Build history of the part. All positions in model axes, mm. Face numbers are marked on the shaded views. A direction names the side the tool comes from. Coordinates: 2 decimals unless noted, no trailing zeros. Order: outer loops, then holes, each group sorted by start corner. A loop starts at its lowest first (then second) coordinate and runs counter-clockwise, first axis right, second up. Notation, with made-up numbers: (64.25, 89.25) -> (90.25, 89.25) arc R29 cw to (90.25, 112.25) -> close; hole circle Ø4 at (35, 62.25). An arc over 180 degrees is marked (long way). Write each question's results on one line, items separated by ' | '.
from build123d import *

# Parameters (mm, degrees)
SKETCH1_R           = 11
BOSS_EXTRUDE1_DEPTH = 55
BOSS_EXTRUDE2_DEPTH = 100
FILLET1_R           = 3


with BuildPart() as part:
    # Sketch1 → Boss-Extrude1 (new body)
    with BuildSketch(Plane(origin=(0, 0, 0), x_dir=(1, 0, 0), z_dir=(0, 1, 0))):
        with Locations(Location((0, 0, 0), (0, 0, 270))):
            Circle(SKETCH1_R)
    extrude(amount=BOSS_EXTRUDE1_DEPTH)

    # Sketch2 → Boss-Extrude2 (add, symmetric)
    with BuildSketch(Plane.XY):
        with BuildLine():
            Line((16, 55), (-16, 55))
            Line((-16, 55), (-16, 60))
            ThreePointArc((-16, 60), (-26.796302084, 77.378878097), (-21, 97))
            ThreePointArc((-21, 97), (-9.389178352, 71.610821648), (16, 60))
            Line((16, 60), (16, 55))
        make_face()
    extrude(amount=BOSS_EXTRUDE2_DEPTH, both=True)

    # Fillet1
    fillet1_edges = [part.edges().sort_by_distance(p)[0] for p in [
        (16, 60, 0),
        (-16, 60, 0),
    ]]
    fillet(fillet1_edges, radius=FILLET1_R)


solid = part.part
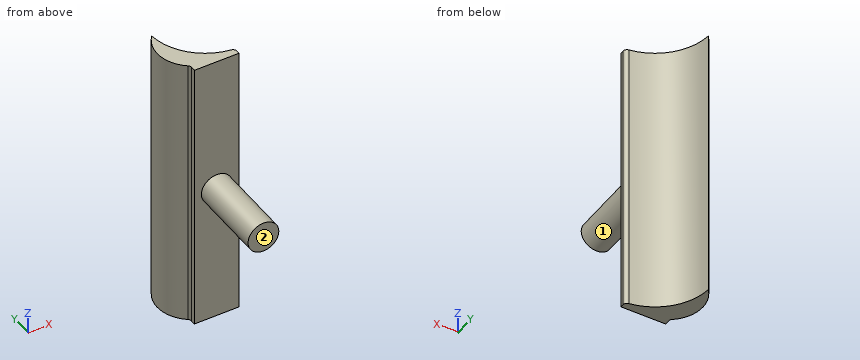
Item 1: Slice it at A-A, the plane z = 83. List the corners of the cut face in (x, y), and give its area (3 significant figures).
Answer:
outline: (-21, 97) arc R25 ccw to (-17.18, 60.85) arc R3 cw to (-16, 58.46) -> (-16, 55) -> (16, 55) -> (16, 57.3) arc R3 ccw to (13.41, 60.27) arc R40 cw to start | area: 618 mm^2
Item 2: Slice it at B-B, the plane x = 0. List the corners of the cut face in (y, z).
Answer:
outline: (0, -11) -> (55, -11) -> (55, -100) -> (64.64, -100) -> (64.64, 100) -> (55, 100) -> (55, 11) -> (0, 11) -> close
Item 3: Drill centre lines: line 1 (Z direction, x = -0.5, y = 32); line 2 (X direction, y = 55.5, z = 62); line 3 (X direction, y = 63, z = -57). Where is each one in solid material? Low to high. Write a range as from..to.
Answer:
line 1: z = -10.99..10.99 | line 2: x = -16..16 | line 3: x = -19.65..3.44
Item 4: Pin check, flat tips, straight feed: pin 1 (10 mm diameter, centred on x = -9.5, y = 49, fed in from +Z); pin 2 (3 mm diameter, centred on y = 56, z = 2, fed in from -X); pin 3 (6 mm diameter, centred on y = 38, z = 4, fed in from -X). Stop position of each tip, or through.
Answer:
pin 1: stops at z = 10.04 | pin 2: stops at x = -16 | pin 3: stops at x = -10.95
Item 5: Tool access for the marked faces 1 and 2: list every direction of +Z, -Z, +X, -X, +Y, -Y with a clear straight run to the whole face (end or side of a thin tool).
Answer:
face 1: -Y | face 2: +Z, -Z, +X, -X, -Y
Item 6: Slice it at C-C, the plane y = 13.5. List the corners of the cut face in (x, z).
Answer:
outline: circle Ø22 at (0, 0)
Item 7: Slice it at D-D, the plane z = 0. List the corners of the cut face in (x, y), and give its area (3 significant figures).
Answer:
outline: (-21, 97) arc R25 ccw to (-17.18, 60.85) arc R3 cw to (-16, 58.46) -> (-16, 55) -> (-11, 55) -> (-11, 0) -> (11, 0) -> (11, 55) -> (16, 55) -> (16, 57.3) arc R3 ccw to (13.41, 60.27) arc R40 cw to start | area: 1,830 mm^2
